```python
from build123d import *

# Parameters (mm, degrees)
F1_DEPTH = 63.5
F0_W     = 25.4670892687
F0_H     = 21.7436235398
F2_DEPTH = 25.4
F3_DEPTH = 7.9375
F5_R     = 5.08


with BuildPart() as f1:
    # F0 (on Front) → F1 (new body, symmetric)
    with BuildSketch(Plane.XZ):
        Polygon((52.4020902812, -17.1774495393), (52.4020902812, 17.1774495393), (30.6584667414, 17.1774495393), (-52.4020902812, 17.1774495393), (-52.4020902812, -17.1774495393), align=None)
    extrude(amount=F1_DEPTH, both=True)

    # F0 (on Front) → F2 (join, symmetric)
    with BuildSketch(Plane.XZ):
        with BuildLine():
            Line((30.6584667414, 17.1774495393), (52.4020902812, 17.1774495393))
            Line((52.4020902812, 17.1774495393), (52.4020902812, 43.2697720826))
            ThreePointArc((52.4020902812, 43.2697720826), (55.8411102963, 51.5723008442), (64.1436390579, 55.0113208592))
            Line((64.1436390579, 55.0113208592), (104.1518747807, 55.0113208592))
            Line((104.1518747807, 55.0113208592), (104.1518747807, 76.754944399))
            Line((104.1518747807, 76.754944399), (64.1436390579, 76.754944399))
            ThreePointArc((64.1436390579, 76.754944399), (40.4660466437, 66.9473644967), (30.6584667414, 43.2697720826))
            Line((30.6584667414, 43.2697720826), (30.6584667414, 17.1774495393))
        make_face()
        with Locations((116.885419415, 65.8831326291)):
            Rectangle(F0_W, F0_H)
    extrude(amount=F2_DEPTH, both=True)

    # F0 (on Front) → F3 (join, symmetric)
    with BuildSketch(Plane.XZ):
        with BuildLine():
            Line((-52.4020902812, 17.1774495393), (30.6584667414, 17.1774495393))
            Line((30.6584667414, 17.1774495393), (30.6584667414, 43.2697720826))
            ThreePointArc((30.6584667414, 43.2697720826), (40.4660466437, 66.9473644967), (64.1436390579, 76.754944399))
            add(Edge.make_bspline(
                [(-52.4020902812, 17.1774495393), (-51.5323504806, 54.1415736079), (24.5702583343, 77.6246711612), (64.1436390579, 76.754944399)],
                knots=[0, 0, 0, 0, 130.8907365743, 130.8907365743, 130.8907365743, 130.8907365743], degree=3))
        make_face()
    extrude(amount=F3_DEPTH, both=True)

    # F0 (on Front) → F4 (revolve)
    with BuildSketch(Plane.XZ):
        Polygon((129.6189640493, 76.754944399), (129.6189640493, 55.0113208592), (129.6189640493, 29.353864491), (154.5970141888, 29.353864491), (154.5970141888, 86.7569819093), (129.6189640493, 86.7569819093), align=None)
    revolve(axis=Axis((129.6189640493, 0, 58.0554232001), (0, 0, -1)))

    # F5
    f5_edges = [f1.edges().sort_by_distance(p)[0] for p in [
        (-52.40209, -63.5, 0),
        (52.40209, -63.5, 0),
        (52.40209, 63.5, 0),
        (-52.40209, 63.5, 0),
    ]]
    fillet(f5_edges, radius=F5_R)


solid = f1.part
```
Input: part model. Units: mm. Frame: model coordinates. A direction names the side the tool comes from. Give positions to 0.01 mm unless a question says otherwise; leave off trailing zeros. Order: outer loops, then holes, each group sorted by start corner. A loop starts at its lowest first (then second) coordinate and runs counter-clockwise, first axis right, second up. Notation, with made-up numbers: M 72.5,45 L 107.5,45 A25 cw 107.5,58 Z; hole C 50.25,14 d2. An arc over 180 degrees is marked long. One line per question, with ' | ' between items. Start each with the question number.
1. First-contact query: pin 1 Ø8 at (y, z) = (-50.5, -4.5) entering from +X; pin 2 Ø16.5 at (x, y) = (0, -46.5) entering from +Z; pin 3 Ø8.5 at (y, z) = (14.5, 35.5) entering from -X. Flat tips, straight axial feed; report the tip coordinate or a pass-through.
2. Access query for faces 1 (the face through (68, -25.4, 61)), 2 (the face through (1, 35, 17.177)), 3 (the face through (30.658, -17, 30)). Directions: +Z, -Z, +X, -X, +Y, -Y. A direction counts if a zero-diameter tool reaches every point of the face in a straight line with its end or side. Return the directions, or none.
3. Material intervals for probe 1 along Z at (x, y) = (26.5, -45); probe 2 along Y at (x, z) = (32, 71); probe 3 along X at (y, z) = (0, 53), sorted ascending. Write a range as [from, to].
4. Section query B-B (x = 107). Return the cut outline in (y, z).
5. Section query C-C (y = 42.5). Return the cut outline in (x, z).
6. Pull-direction query (X, two-part tool) for faces 4 (the face through (55.75, -0.36, 51.48)), 5 (the face through (153.444, -7.503, 58.457)), 6 (the face through (130, 0, 29.354)), 7 (the face through (-50.953, -61.972, -0.24)); classes: released by +X, released by -X, zero draft, split by the parting line, or undercut.
7. Section query A-A (y = -15.5). Return the cut outline in (x, z).
8. Section query D-D (x = 141). Return the cut outline in (y, z).
Here are the results:
1) pin 1: x = 52.4 | pin 2: z = 17.18 | pin 3: x = 30.66
2) face 1: +Z, +X, -X, -Y | face 2: +Z, -X, +Y | face 3: +Z, -X, -Y
3) probe 1: [-17.18, 17.18] | probe 2: [-7.94, 7.94] | probe 3: [-24.75, 57.57], [104.64, 154.6]
4) outline: M -25.4,55.01 L -10.6,55.01 L -10.6,29.35 L 10.6,29.35 L 10.6,55.01 L 25.4,55.01 L 25.4,76.75 L 10.6,76.75 L 10.6,86.76 L -10.6,86.76 L -10.6,76.75 L -25.4,76.75 Z
5) outline: M -52.4,-17.18 L 52.4,-17.18 L 52.4,17.18 L -52.4,17.18 Z
6) face 4: undercut | face 5: undercut | face 6: zero draft | face 7: released by -X
7) outline: M -52.4,-17.18 L 52.4,-17.18 L 52.4,43.27 A11.74 cw 64.14,55.01 L 110.03,55.01 L 110.03,29.35 L 149.21,29.35 L 149.21,86.76 L 110.03,86.76 L 110.03,76.75 L 64.14,76.75 A33.49 ccw 30.66,43.27 L 30.66,17.18 L -52.4,17.18 Z
8) outline: M -22.23,29.35 L 22.23,29.35 L 22.23,86.76 L -22.23,86.76 Z
